The figure shows three views and two pictorial views of one solid part (mm, origin at its lowest corner). Answer the questions. Give positions to 0.01 mm unless a question says otherwise; leave off trailing zeros. Loops run counter-clockwise (first coordinate to the right, second up) from the corner with the lowest first, then second, coordinate; pieces in that order, holes last. Notation, with made-up numbers: (-36.75, -1) - (18.25, -1) arc R34 ccw to (18.25, 38) - close; hole circle Ø1 at (61, -13.5). An arc over 180 degrees is marked (long way). Use a Markdown table: item, result. Add a question column.
Item 1: A cutting plane is placed at B-B (x = 0.95). Determine the outline of the cut face in (y, z) (3 decimals), plus the area to 4 significant figures.
Item 2: Consider probe 1 along X at (y, z) = (6.6, 0.75); probe 2 along Y at (x, z) = (27.75, 0.2) (3 decimals). Determine where each line is inside the solid, lowest interval first. Write a range as [from, to].
Item 3: A cutting plane is placed at A-A (y = 11.6). Determine the outline of the cut face in (x, z) (3 decimals), plus the area to 4 significant figures.
Item 4: Each of these flat-tipped pins is pushed along its axis until it touches: P1, Ø0.6, axis at x = 27.5, y = 7, coming from the -Z side; P2, Ø1.5, axis at x = 0.95, y = 6.6, coming from the +Z side. Where does it stop, or does it pass through?
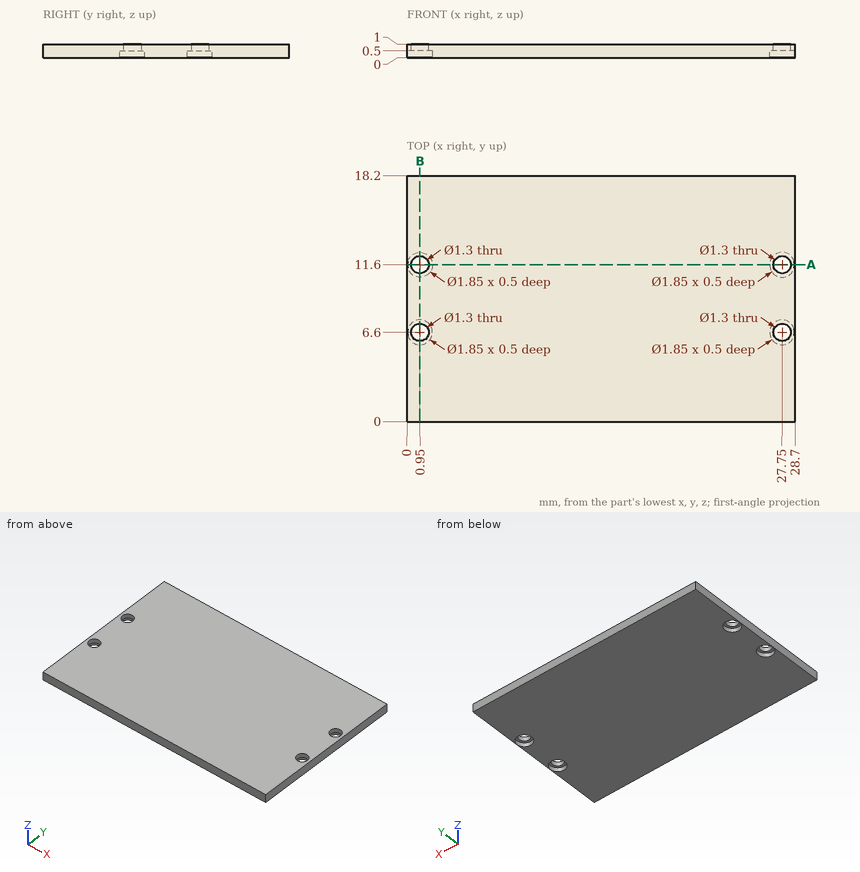
Geometry says:
| question | item | result |
|---|---|---|
| 1 | outline | (0, 0) - (5.675, 0) - (5.675, 0.5) - (5.95, 0.5) - (5.95, 1) - (0, 1) - close; (7.25, 0.5) - (7.525, 0.5) - (7.525, 0) - (10.675, 0) - (10.675, 0.5) - (10.95, 0.5) - (10.95, 1) - (7.25, 1) - close; (12.25, 0.5) - (12.525, 0.5) - (12.525, 0) - (18.2, 0) - (18.2, 1) - (12.25, 1) - close |
| 1 | area | 15.05 mm² |
| 2 | probe 1 | [0, 0.3], [1.6, 27.1], [28.4, 28.7] |
| 2 | probe 2 | [0, 5.675], [7.525, 10.675], [12.525, 18.2] |
| 3 | outline | (0, 0) - (0.025, 0) - (0.025, 0.5) - (0.3, 0.5) - (0.3, 1) - (0, 1) - close; (1.6, 0.5) - (1.875, 0.5) - (1.875, 0) - (26.825, 0) - (26.825, 0.5) - (27.1, 0.5) - (27.1, 1) - (1.6, 1) - close; (28.4, 0.5) - (28.675, 0.5) - (28.675, 0) - (28.7, 0) - (28.7, 1) - (28.4, 1) - close |
| 3 | area | 25.55 mm² |
| 4 | P1 | z = 0.5 |
| 4 | P2 | z = 1 |
